Input: part model. Units: mm. Frame: model coordinates. Face numbers are marked on the shaded views. Give positions to 0.01 mm unless a question says otherwise; leave off trailing zeros. Loops run counter-clockwise (first coordinate to the right, second up) from the corner with the lowest first, then second, coordinate; pieces in that order, holes last. Notation, with made-up numbers: (-34, 20) -> (-11, 20) arc R29 ccw to (-11, 56) -> close; hole circle Ø7 at (1.25, 77). An arc over 180 degrees is marked (long way). Answer as a JSON object with one key per item and string values. Group by question number.
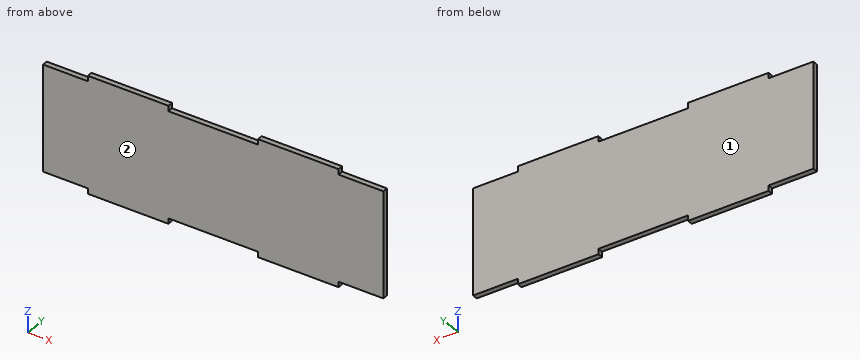
```python
from build123d import *

# Parameters (mm, degrees)
SKETCH1_W               = 190
SKETCH1_H               = 65
BOSS_EXTRUDE1_DEPTH     = 3
CUT_EXTRUDE1_DEPTH      = 101.450236436
CUT_EXTRUDE1_DEPTH_BACK = 3
SKETCH2_OUTSIDE_W       = 232.166
SKETCH2_OUTSIDE_H       = 107.166


with BuildPart() as part:
    # Sketch1 → Boss-Extrude1 (new body)
    with BuildSketch(Plane(origin=(0, 0, 0), x_dir=(1, 0, 0), z_dir=(0, 1, 0))):
        Rectangle(SKETCH1_W, SKETCH1_H)
    extrude(amount=BOSS_EXTRUDE1_DEPTH)

    # Sketch2 outside → Cut-Extrude1 (cut, two sides: drawn at the far end of the back side and taken through both)
    with BuildSketch(Plane(origin=(0, 3, 0), x_dir=(1, 0, 0), z_dir=(0, 1, 0)).offset(-CUT_EXTRUDE1_DEPTH_BACK)):
        Rectangle(SKETCH2_OUTSIDE_W, SKETCH2_OUTSIDE_H)
        Polygon((-95, 29.5), (-70, 29.5), (-70, 32.5), (-25, 32.5), (-25, 29.5), (25, 29.5), (25, 32.5), (70, 32.5), (70, 29.5), (95, 29.5), (95, -29.5), (70, -29.5), (70, -32.5), (25, -32.5), (25, -29.5), (-25, -29.5), (-25, -32.5), (-70, -32.5), (-70, -29.5), (-95, -29.5), align=None, mode=Mode.SUBTRACT)
    extrude(amount=CUT_EXTRUDE1_DEPTH + CUT_EXTRUDE1_DEPTH_BACK, mode=Mode.SUBTRACT)


solid = part.part
```
Q1. Pin query (flat end, axial travel): pin 1 Ø1 at (x, y) = (12, 1.5) entering from -Z; pin 2 Ø0.9 at (y, z) = (1, -30.5) entering from -X; pin 3 Ø1.5 at (x, y) = (88, 1) entering from +Z. Return the tip coordinate at first contact, or that it passes through.
Q2. Section B-B on x = 0.5. Return the cut outline in (y, z).
Q3. Section A-A on y = 1.6. Return the cut outline in (x, z), then the cut area to 4 significant figures.
Q4. Pull-direction query (Y, two-part tool) for the marked faces 1 and 2; classes: +Y half, -Y half, draft (parallel to the pull), parting line (faces both ways), or undercut.
Q5. Ray query, probe 1 along Z at (x, y) = (14.5, 2.8). Return the intervals inside material, ascending.
Numbers:
{
 "1": {"pin 1": "stops at z = -29.5", "pin 2": "stops at x = -70", "pin 3": "stops at z = 29.5"},
 "2": {"outline": "(0, -29.5) -> (3, -29.5) -> (3, 29.5) -> (0, 29.5) -> close"},
 "3": {"outline": "(-95, -29.5) -> (-70, -29.5) -> (-70, -32.5) -> (-25, -32.5) -> (-25, -29.5) -> (25, -29.5) -> (25, -32.5) -> (70, -32.5) -> (70, -29.5) -> (95, -29.5) -> (95, 29.5) -> (70, 29.5) -> (70, 32.5) -> (25, 32.5) -> (25, 29.5) -> (-25, 29.5) -> (-25, 32.5) -> (-70, 32.5) -> (-70, 29.5) -> (-95, 29.5) -> close", "area": "11,750 mm²"},
 "4": {"face 1": "+Y half", "face 2": "-Y half"},
 "5": {"probe 1": "z = -29.5 to 29.5"}
}
